```python
from build123d import *

# Parameters (mm, degrees)
ESBO_O1_W                = 60
ESBO_O1_H                = 60
ESBO_O1_R                = 29
RESSALTO_EXTRUS_O1_DEPTH = 15
ESBO_O2_R                = 2
CORTE_EXTRUS_O1_DEPTH    = 15
ESBO_O3_R                = 3.5
CORTE_EXTRUS_O2_DEPTH    = 5
FILETE1_R                = 5
RESSALTO_EXTRUS_O2_DEPTH = 2
ESBO_O5_R                = 3.5
RESSALTO_EXTRUS_O3_DEPTH = 9
ESBO_O6_R                = 1.5
CORTE_EXTRUS_O3_DEPTH    = 18.3
ESBO_O7_R                = 2.5
CORTE_EXTRUS_O4_DEPTH    = 1.5


with BuildPart() as part:
    # Esboço1 → Ressalto-extrusão1 (new body)
    with BuildSketch(Plane.XY):
        with Locations((30, 30)):
            Rectangle(ESBO_O1_W, ESBO_O1_H)
        with Locations((30, 30)):
            Circle(ESBO_O1_R, mode=Mode.SUBTRACT)
    extrude(amount=RESSALTO_EXTRUS_O1_DEPTH)

    # Esboço2 → Corte-extrusão1 (cut)
    with BuildSketch(Plane.XY.offset(15)):
        with Locations((5, 55)):
            Circle(ESBO_O2_R)
        with Locations((55, 55)):
            Circle(ESBO_O2_R)
        with Locations((55, 5)):
            Circle(ESBO_O2_R)
        with Locations((5, 5)):
            Circle(ESBO_O2_R)
    extrude(amount=-CORTE_EXTRUS_O1_DEPTH, mode=Mode.SUBTRACT)

    # Esboço3 → Corte-extrusão2 (cut)
    with BuildSketch(Plane.XY.offset(15)):
        with Locations((5, 55)):
            Circle(ESBO_O3_R)
        with Locations((55, 55)):
            Circle(ESBO_O3_R)
        with Locations((55, 5)):
            Circle(ESBO_O3_R)
        with Locations((5, 5)):
            Circle(ESBO_O3_R)
    extrude(amount=-CORTE_EXTRUS_O2_DEPTH, mode=Mode.SUBTRACT)

    # Filete1
    filete1_edges = [part.edges().sort_by_distance(p)[0] for p in [
        (0, 60, 7.5),
        (60, 60, 7.5),
        (60, 0, 7.5),
        (0, 0, 7.5),
    ]]
    fillet(filete1_edges, radius=FILETE1_R)

    # Esboço4 → Ressalto-extrusão2 (add)
    with BuildSketch(Plane(origin=(0, 0, 0), x_dir=(-1, 0, 0), z_dir=(0, 0, -1))):
        with BuildLine():
            Line((-30.130751647, 45.999465741), (-48.233254252, 52.551018589))
            ThreePointArc((-48.233254252, 52.551018589), (-49.721988735, 51.261306647), (-51.119742067, 49.873512398))
            Line((-51.119742067, 49.873512398), (-36.546722488, 44.599329596))
            ThreePointArc((-36.546722488, 44.599329596), (-43.465751902, 38.641384479), (-45.999465741, 29.869248353))
            Line((-45.999465741, 29.869248353), (-52.551018589, 11.766745748))
            ThreePointArc((-52.551018589, 11.766745748), (-51.261306647, 10.278011265), (-49.873512398, 8.880257933))
            Line((-49.873512398, 8.880257933), (-44.599329596, 23.453277512))
            ThreePointArc((-44.599329596, 23.453277512), (-38.641384479, 16.534248098), (-29.869248353, 14.000534259))
            Line((-29.869248353, 14.000534259), (-11.766745748, 7.448981411))
            ThreePointArc((-11.766745748, 7.448981411), (-10.278011265, 8.738693353), (-8.880257933, 10.126487602))
            Line((-8.880257933, 10.126487602), (-23.453277512, 15.400670404))
            ThreePointArc((-23.453277512, 15.400670404), (-16.534248098, 21.358615521), (-14.000534259, 30.130751647))
            Line((-14.000534259, 30.130751647), (-7.448981411, 48.233254252))
            ThreePointArc((-7.448981411, 48.233254252), (-8.738693353, 49.721988735), (-10.126487602, 51.119742067))
            Line((-10.126487602, 51.119742067), (-15.400670404, 36.546722488))
            ThreePointArc((-15.400670404, 36.546722488), (-21.358615521, 43.465751902), (-30.130751647, 45.999465741))
        make_face()
    extrude(amount=-RESSALTO_EXTRUS_O2_DEPTH)

    # Esboço5 → Ressalto-extrusão3 (add)
    with BuildSketch(Plane.XY.offset(2)):
        with Locations((30, 30)):
            Circle(ESBO_O5_R)
    extrude(amount=RESSALTO_EXTRUS_O3_DEPTH)

    # Esboço6 → Corte-extrusão3 (cut)
    with BuildSketch(Plane.XY.offset(11)):
        with Locations((30, 30)):
            Circle(ESBO_O6_R)
    extrude(amount=-CORTE_EXTRUS_O3_DEPTH, mode=Mode.SUBTRACT)

    # Esboço7 → Corte-extrusão4 (cut)
    with BuildSketch(Plane(origin=(0, 0, 0), x_dir=(-1, 0, 0), z_dir=(0, 0, -1))):
        with Locations((-30, 30)):
            Circle(ESBO_O7_R)
    extrude(amount=-CORTE_EXTRUS_O4_DEPTH, mode=Mode.SUBTRACT)


solid = part.part
```
CAD build for the part. Positions are in the model's coordinates, mm. A direction names the side the tool comes from. Round coordinates to 2 decimals unless told otherwise and drop trailing zeros. Loops run counter-clockwise (first coordinate to the right, second up) from the corner with the lowest first, then second, coordinate; pieces in that order, holes last. Notation, with made-up numbers: M -14,80 L -10,80 A6 cw -10,85 Z; hole C 55.5,71 d2. An arc over 180 degrees is marked long. Use a Markdown table: item, result. Add a question column.
(1) Drill centre lines: line 1 (X direction, y = 30.5, z = 7.5); line 2 (Y direction, x = 34, z = 1); line 3 (Z direction, x = 17.5, y = 21). Where is each one in solid material? Low to high.
(2) Cut at B-B (z = 12.5). Give the cut face in (x, y).
(3) Pull direction X, two halves, no side cores. Call faces 1 (the face through (60, 30, 7)), 2 (the face through (1, 58, 8)), 3 (the face through (38.75, 16.605, 0.986)): +X half, -X half, draft (parallel to the pull), parting line (faces both ways), or undercut.
(4) Cut at A-A (z = 9). Give the cut face in (x, y), and give its area (3 significant figures).
(5) Which spindle directions (+Z, -Z, +X, -X, +Y, -Y) get a long thin tool onto all of the face, cutting with end or side? Do faces 4 (the face through (28, 30, 1.5)), 5 (the face through (58, 1, 8)), 6 (the face through (39.06, 49.23, 0.99)), 7 (the face through (29.54, 33.47, 6.44)). Say none if no direction does.
(6) Cut at D-D (y = 49). Give the cut face in (x, z), and give its area (3 significant figures).
(7) Cut at C-C (x = 17.5). Give the cut face in (y, z).
(8) Flat gauge pins, fed straight in: pin 1 (3 mm diameter, centred on x = 5, y = 55, fed in from +Z); pin 2 (4 mm diameter, centred on x = 30, y = 30, fed in from +Z); pin 3 (4 mm diameter, centred on x = 30, y = 30, fed in from -Z); pin 4 (6.5 mm diameter, centred on x = 55, y = 55, fed in from +Z). Where does each tip first touch, or does it go through?
Geometry says:
| question | item | result |
|---|---|---|
| 1 | line 1 | x = 0 to 1, 26.54 to 28.59, 31.41 to 33.46, 59 to 60 |
| 1 | line 2 | y = 0 to 1.28, 14.51 to 47.4, 58.72 to 60 |
| 1 | line 3 | z = 0 to 2 |
| 2 | outline | M 0,5 A5 ccw 5,0 L 55,0 A5 ccw 60,5 L 60,55 A5 ccw 55,60 L 5,60 A5 ccw 0,55 Z; hole C 30,30 d58; hole C 5,5 d7; hole C 5,55 d7; hole C 55,5 d7; hole C 55,55 d7 |
| 3 | face 1 | +X half |
| 3 | face 2 | -X half |
| 3 | face 3 | undercut |
| 4 | outline | M 0,5 A5 ccw 5,0 L 55,0 A5 ccw 60,5 L 60,55 A5 ccw 55,60 L 5,60 A5 ccw 0,55 Z; C 30,30 d7; hole C 30,30 d58; hole C 5,5 d4; hole C 5,55 d4; hole C 30,30 d3; hole C 55,5 d4; hole C 55,55 d4 |
| 4 | area | 918 mm² |
| 5 | face 4 | -Z |
| 5 | face 5 | +Z, -Z, +X, -Y |
| 5 | face 6 | +Z, -Z |
| 5 | face 7 | +Z |
| 6 | outline | M 0,0 L 10.89,0 L 10.89,2 L 8.09,2 L 8.09,15 L 0,15 Z; M 38.42,0 L 48.71,0 L 48.71,2 L 38.42,2 Z; M 51.91,0 L 60,0 L 60,15 L 51.91,15 Z |
| 6 | area | 269 mm² |
| 7 | outline | M 0,0 L 3.83,0 L 3.83,15 L 0,15 Z; M 9.52,0 L 13.25,0 L 13.25,2 L 9.52,2 Z; M 20.01,0 L 39.99,0 L 39.99,2 L 20.01,2 Z; M 56.17,0 L 60,0 L 60,15 L 56.17,15 Z |
| 8 | pin 1 | passes through |
| 8 | pin 2 | stops at z = 11 |
| 8 | pin 3 | stops at z = 1.5 |
| 8 | pin 4 | stops at z = 10 |
